Source: three-view drawing plus pictorial views. Frame: mm from the lowest corner of the part. A direction names the side the tool comes from. Coordinates: 2 decimals unless noted, no trailing zeros. Write each loop counter-clockwise with the first axis right and the second up, starting at its lowest first coordinate (ties: lowest second). Pieces come first, ordered by that corner, then holes. Notation, with made-up numbers: M -6.75,4.25 L 20.25,4.25 A21 ccw 20.25,26.25 Z; hole C -29,-14.75 d6. An arc over 180 degrees is marked long. Use CSV: the item, a comma, the result in double quotes.
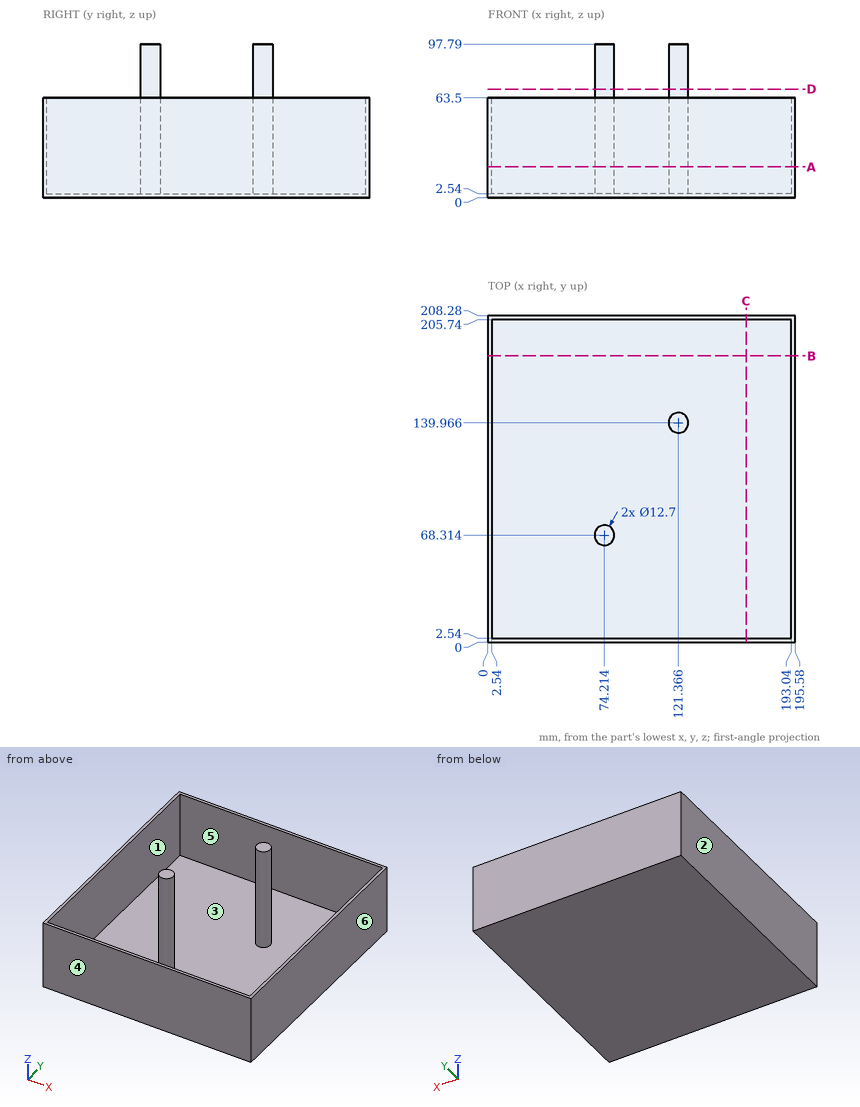
1. Mould query, pull axis X, two halves, no side actions, for the marked faces 1, 2, 3 and 4. Classes: pulls with the +X half, pulls with the -X half, needs draft (parallel to the pull), parting line crosses it, or undercut.
Resolved:
face 1,"undercut"
face 2,"pulls with the -X half"
face 3,"undercut"
face 4,"needs draft"
2. Access query for the marked faces 5 and 6. Directions: +Z, -Z, +X, -X, +Y, -Y. A direction counts if a zero-diameter tool reaches every point of the face in a straight line with its end or side. Return the directions, or none.
Resolved:
face 5,"+Z"
face 6,"+Z, -Z, +X, +Y, -Y"
3. Section C-C (x = 164.5). Return loops of the section in (y, z).
Resolved:
outline,"M 0,0 L 208.28,0 L 208.28,63.5 L 205.74,63.5 L 205.74,2.54 L 2.54,2.54 L 2.54,63.5 L 0,63.5 Z"
4. Contact query for flat-ended pins moving along their axis: pin 1 Ø3 at (x, y) = (111, 135) entering from -Z; pin 2 Ø10 at (x, y) = (112, 98) entering from +Z. Output: stop coordinate, or through.
Resolved:
pin 1,"stops at z = 0"
pin 2,"stops at z = 2.54"
5. Section D-D (z = 69). Return loops of the section in (x, y), then the cut area to 3 significant figures.
Resolved:
outline,"C 74.21,68.31 d12.7; C 121.37,139.97 d12.7"
area,"253 mm^2"
6. Section B-B (y = 182.5). Return loops of the section in (x, z).
Resolved:
outline,"M 0,0 L 195.58,0 L 195.58,63.5 L 193.04,63.5 L 193.04,2.54 L 2.54,2.54 L 2.54,63.5 L 0,63.5 Z"
7. Material intervals for line 1 (X direction, y = 149, z = 26.5); line 2 (Y direction, x = 171, z = 6); line 3 (Y direction, x = 117, z = 26.5) (1 decimal), sorted ascending. Write a range as [from, to].
Resolved:
line 1,"x = [0, 2.54], [193.04, 195.58]"
line 2,"y = [0, 2.54], [205.74, 208.28]"
line 3,"y = [0, 2.5], [135.4, 144.6], [205.7, 208.3]"
8. Section A-A (z = 19.5). Return loops of the section in (x, y), then the cut area to 3 significant figures.
Resolved:
outline,"M 0,0 L 195.58,0 L 195.58,208.28 L 0,208.28 Z; C 74.21,68.31 d12.7; C 121.37,139.97 d12.7; hole M 2.54,2.54 L 193.04,2.54 L 193.04,205.74 L 2.54,205.74 Z"
area,"2,280 mm^2"
